Autodesk Inventor part; units mm, degrees
ref_plane "YZ Plane" through (0, 0, 0) normal (1, 0, 0) x (0, 1, 0)
ref_plane "XZ Plane" through (0, 0, 0) normal (0, 1, 0) x (-1, 0, 0)
ref_plane "XY Plane" through (0, 0, 0) normal (0, 0, 1) x (1, 0, 0)
sketch "Sketch1" plane through (0, 0, 0) normal (0, 0, 1) x (1, 0, 0)
  circle A0 centre (0, 0) radius 6.3309
  dimension "d0" = 12.6619
extrude "Extrusion1" add sketch "Sketch1" against normal blind 60.0964
sketch "Sketch2" plane through (0, 0, 0) normal (0, 1, 0) x (-1, 0, 0)
  line L0 (-6.3309, -60.0964) -> (-6.3309, 0)
  line L1 (-6.3309, 0) -> (6.3309, 0)
  line L2 (6.3309, 0) -> (6.3309, -60.0964)
  line L3 (6.3309, -60.0964) -> (-6.3309, -60.0964)
  line L4 (6.3309, -12.573) -> (-6.3309, -12.573)
  point P0 (0, 0)
  dimension "d3" = 12.573
extrude "Extrusion2" cut sketch "Sketch2" along normal mid plane 4.9403 contours L0 L1 L2 L4
sketch "Sketch3" plane through (0, 2.4702, 0) normal (0, -1, 0) x (1, 0, 0)
  line L0 (-5.8292, 0) -> (5.8292, 0) construction
  line L1 (5.8292, 0) -> (5.8292, -12.573) construction
  line L2 (-5.8292, -12.573) -> (5.8292, -12.573) construction
  line L3 (-5.8292, -60.0964) -> (-5.8292, -12.573) construction
  line L4 (5.8292, -60.0964) -> (-5.8292, -60.0964) construction
  line L5 (5.8292, -12.573) -> (5.8292, -60.0964) construction
  line L6 (-5.8292, -12.573) -> (-5.8292, 0) construction
  line L7 (0, 0) -> (0, -12.573) construction
  circle A0 centre (0, -4.064) radius 1.651
  dimension "d6" = 3.302
  dimension "d7" = 4.064
extrude "Extrusion3" cut sketch "Sketch3" along normal through all both and the other way through all
sketch "Sketch4" plane through (0, 0, 0) normal (0, 1, 0) x (-1, 0, 0)
  line L0 (-6.3309, -12.573) -> (6.3309, -12.573)
  line L1 (6.3309, -12.573) -> (6.3309, -60.0964)
  line L2 (6.3309, -60.0964) -> (-6.3309, -60.0964)
  line L3 (-6.3309, -60.0964) -> (-6.3309, -12.573)
  line L4 (0, -60.0964) -> (0, -48.5629) construction
  line L5 (6.3309, -49.911) -> (0.3196, -59.9156)
  arc A0 (0, -60.0964) -> (0.3196, -59.9156) centre (0, -59.7236) ccw
  line L6 (0, -72.1662) -> (0, 12.0277)
  point P0 (0, 0)
  dimension "d10" = 10.1854
  dimension "d11" = 31
revolve "Revolution1" cut sketch "Sketch4" angle 360 about axis through (0, 0, -10) along (0, 0, 1) contours A0 L5 L1 L2
fillet "Fillet1" radius 0.0762 2 edges at (0, -6.3309, -49.911) (0, 6.3309, -49.911)
fillet "Fillet2" radius 0.127 2 edges at (0, -6.3309, 0) (0, 6.3309, 0)
chamfer "Chamfer1" distance 0.127 angle 45 2 edges at (-1.651, -6.1119, -4.0553) (-1.651, 6.1119, -4.0553)
properties part number "solenoid pin"
Source: CAD feature listing. Evaluate the final solid. Frame: model axes, mm. A direction names the side the tool comes from. Coordinates: 2 decimals unless noted, no trailing zeros. Loops run counter-clockwise (first coordinate to the right, second up) from the corner with the lowest first, then second, coordinate; pieces in that order, holes last. Notation, with made-up numbers: (-7.75, 69) -> (35.25, 69) arc R20 ccw to (35.25, 80) -> close; hole circle Ø4 at (8, 23). An arc over 180 degrees is marked (long way). One line per item, written item: value. Start each with the question number.
Q1. Contact query for flat-ended pins moving along their axis: P1, Ø1, axis at y = 2.5, z = -7.5, coming from the -X side; P2, Ø3, axis at y = 3.5, z = -42.5, coming from the +X side; P3, Ø2.5, axis at x = 0, z = -4.064, coming from the -Y side; P4, Ø2, axis at x = 1.5, z = -29.5, coming from the +Y side. Output: stop coordinate, or through.
Q2. Section query B-B, the plane z = -5. Give the number of separate pieces and of enclosed holes in the cut face, and give its area (3 significant figures).
Q3. Set-up query: faces 4 (the face through (-5.024, -3.852, -24.66)), 5 (the face through (0, 2.47, -6)). Return all of +Z, -Z, +X, -X, +Y, -Y with unobstructed straight access to the full face (end or side cutting, diameter ignored); none if empty.
Q4. Line query: line 1 along Z through (x, y) = (0.75, -2.75); line 2 along Z through (x, y) = (0, 4.95) (3 decimals); line 3 along Y through (x, z) = (-2, -3.5). Output: solid intervals per line, ascending.
Q5. Section query A-A, the plane z = -32. Return the cut outline in (x, y).
Q6. Mould query, pull axis Y, two halves, no side actions, for faces 1 (the face through (-2.57, -0.81, -55.96)), 2 (the face through (-0.21, -4.31, -5.7)), 3 (the face through (0, 0, -12.573)). Classes: pulls with the +Y half, pulls with the -Y half, needs draft (parallel to the pull), parting line crosses it, or undercut.
Q7. Section query C-C, the plane z = -52. Return the cut outline in (x, y).
Results:
1. P1: x = -5.83
1. P2: x = 6.01
1. P3: through
1. P4: y = 6.31
2. separate pieces: 4
2. enclosed holes: 0
2. area: 44.2 mm^2
3. face 4: +Z, -Z
3. face 5: +Z, +X, -X
4. line 1: -55.7 to -5.53, -2.59 to 0
4. line 2: -52.209 to -5.715, -2.413 to 0
4. line 3: -6.01 to -2.47, 2.47 to 6.01
5. outline: circle Ø12.66 at (0, 0)
6. face 1: parting line crosses it
6. face 2: needs draft
6. face 3: undercut
7. outline: circle Ø10.15 at (0, 0)
